Geometry check sheet. Reference: drawing and pictorial views, mm from the part's lowest x, y, z. Coordinates: 2 decimals unless noted, no trailing zeros. Loops run counter-clockwise (first coordinate to the right, second up) from the corner with the lowest first, then second, coordinate; pieces in that order, holes last. Notation, with made-up numbers: (67.25, -31.5) - (77.25, -31.5) arc R35 ccw to (77.25, 1.5) - close; hole circle Ø10 at (54, 19). An arc over 180 degrees is marked (long way). Use a Markdown table: item, result. Add a question column.
1) Sectioned sample at C-C, the plane x = 2.8. Enter the section's corners in (y, z).
2) Thickness scan on line 1 (X direction, y = 0.6, z = 14); line 2 (X direction, y = 0.75, z = 14.5) (1 decimal); line 3 (Z direction, x = 18.5, y = 0.45) (1 decimal). Record the ranges inside material, lowest first.
3) Sectioned sample at B-B, the plane y = 0.2. State how many separate pieces and enclosed holes the cut face has.
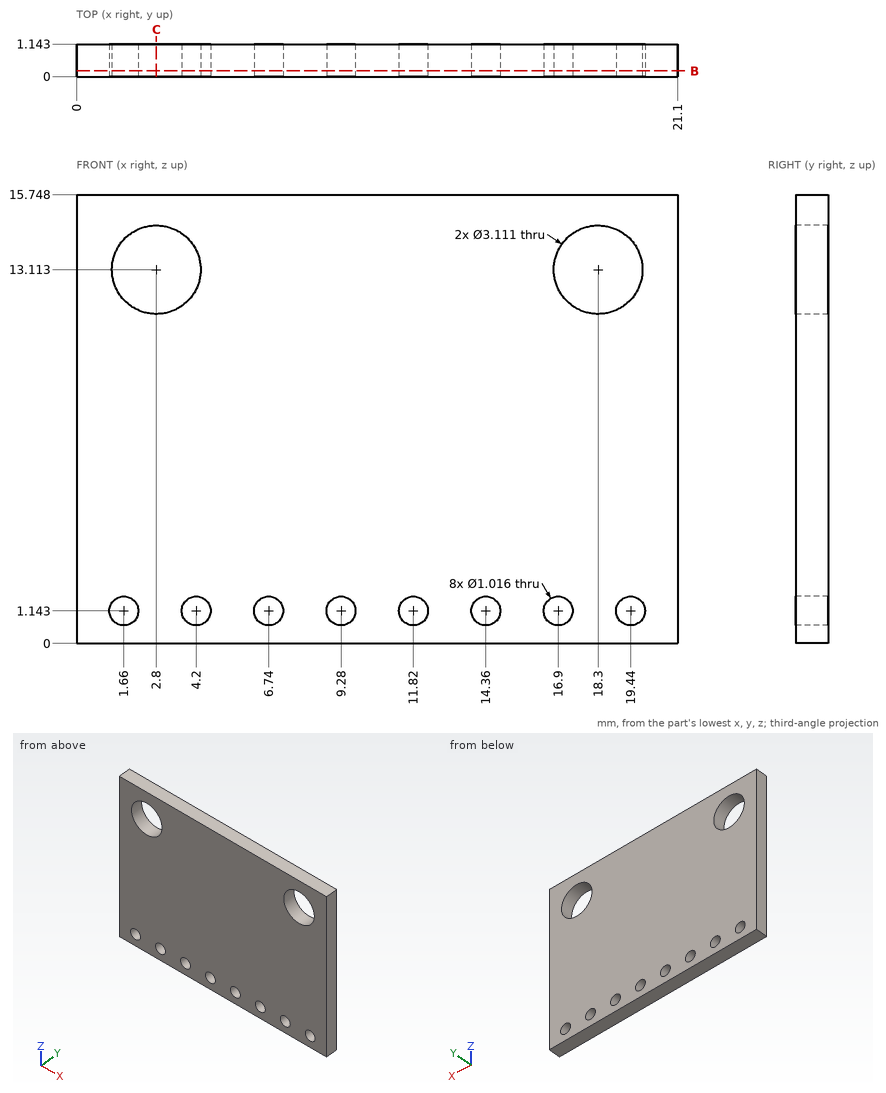
Solved:
| question | item | result |
|---|---|---|
| 1 | outline | (0, 0) - (1.14, 0) - (1.14, 11.56) - (0, 11.56) - close; (0, 14.67) - (1.14, 14.67) - (1.14, 15.75) - (0, 15.75) - close |
| 2 | line 1 | x = 0 to 1.52, 4.08 to 17.02, 19.58 to 21.1 |
| 2 | line 2 | x = 0 to 2.1, 3.5 to 17.6, 19 to 21.1 |
| 2 | line 3 | z = 0 to 11.6, 14.7 to 15.7 |
| 3 | separate pieces | 1 |
| 3 | enclosed holes | 10 |
